Can you work these out from the model? Positions are in its coordinate system, mm. A direction names the side the tool comes from. Coordinates: 2 decimals unless noted, no trailing zeros. Write each loop counter-clockwise with the first axis right and the second up, starting at its lowest first coordinate (ties: lowest second). Pieces come first, ordered by that corner, then holes. Notation, with made-up numbers: M -28.5,55.25 L -12.5,55.25 A20 cw -12.5,59.25 Z; hole C 85,-16.75 d1. An arc over 180 degrees is marked long. Use one line per item in the form item = value. Start each with the question number.
Autodesk Inventor part; units mm, degrees
ref_plane "YZ Plane" through (0, 0, 0) normal (1, 0, 0) x (0, 1, 0)
ref_plane "XZ Plane" through (0, 0, 0) normal (0, 1, 0) x (-1, 0, 0)
ref_plane "XY Plane" through (0, 0, 0) normal (0, 0, 1) x (1, 0, 0)
sketch "Sketch1" plane through (0, 0, 0) normal (0, 1, 0) x (-1, 0, 0)
  line L0 (22, 30) -> (-22, 30)
  line L1 (-22, 30) -> (-22, -30)
  line L2 (-22, -30) -> (22, -30)
  line L3 (22, -30) -> (22, 30)
  line L4 (22, 30) -> (-22, -30) construction
  line L5 (-22, 30) -> (22, -30) construction
  point P0 (0, 0)
  dimension "d0" = 44
  dimension "d1" = 60
extrude "Extrusion1" add sketch "Sketch1" along normal blind 8
sketch "Sketch4" plane through (0, 8, 0) normal (0, 1, 0) x (1, 0, 0)
  circle A0 centre (-17, -24) radius 1.55
  circle A1 centre (17, 24) radius 1.55
  circle A2 centre (17, -24) radius 1.55
  circle A3 centre (-17, 24) radius 1.55
  point P0 (0, 0)
  dimension "d6" = 3.1
  dimension "d7" = 3.1
  dimension "d8" = 3.1
  dimension "d9" = 3.1
  dimension "d10" = 17
  dimension "d11" = 24
  dimension "d12" = 17
  dimension "d13" = 17
  dimension "d14" = 17
  dimension "d15" = 24
  dimension "d16" = 24
  dimension "d17" = 24
hole "Hole1" at (-17, 8, 24) at (-17, 8, -24) at (17, 8, -24) at (17, 8, 24) direction (0, -1, 0) diameter 3.1 depth 8 tip angle 118
sketch "Sketch5" plane through (0, 0, 0) normal (0, -1, 0) x (1, 0, 0)
  line L0 (-12, -18) -> (-22, -18)
  line L1 (-22, -18) -> (-22, -30)
  line L2 (-22, -30) -> (-12, -30)
  line L3 (-12, -30) -> (-12, -18)
  line L4 (22, -18) -> (12, -18)
  line L5 (12, -18) -> (12, -30)
  line L6 (12, -30) -> (22, -30)
  line L7 (22, -30) -> (22, -18)
  line L8 (22, 30) -> (12, 30)
  line L9 (12, 30) -> (12, 18)
  line L10 (12, 18) -> (22, 18)
  line L11 (22, 18) -> (22, 30)
  line L12 (-12, 30) -> (-22, 30)
  line L13 (-22, 30) -> (-22, 18)
  line L14 (-22, 18) -> (-12, 18)
  line L15 (-12, 18) -> (-12, 30)
  line L16 (-22, -30) -> (-22, 30)
  line L17 (22, -30) -> (-22, -30)
  line L18 (22, 30) -> (22, -30)
  line L19 (-22, 30) -> (22, 30)
  point P0 (0, 0)
  dimension "d25" = 10
  dimension "d26" = 12
  dimension "d27" = 10
  dimension "d28" = 12
  dimension "d29" = 10
  dimension "d30" = 12
  dimension "d31" = 10
  dimension "d32" = 12
extrude "Extrusion2" cut sketch "Sketch5" against normal blind 4 contours L3 L2 L1 L0 | L13 L12 L15 L14 | L5 L4 L7 L6 | L8 L11 L10 L9
fillet "Fillet1" radius 3 4 edges at (22, 6, -30) (-22, 6, -30) (22, 6, 30) (-22, 6, 30)
equation "\"d27\" = d25"
equation "\"d28\" = d26"
equation "\"d29\" = d25"
equation "\"d30\" = d26"
equation "\"d31\" = d25"
equation "\"d32\" = d26"
properties part number "motor_driver_support"
1) Will these pins go through, and if not, where does the flat tip stop? pin 1 Ø2 at (y, z) = (2.5, -22.5) entering from +X; pin 2 Ø4.5 at (x, y) = (-19, 1.5) entering from +Z; pin 3 Ø4.5 at (y, z) = (1.5, -22) entering from -X; pin 4 Ø3 at (x, z) = (17, -24) entering from +Y.
2) Suppose I cut it at D-D on x = -14. Please give me the cut outline in (y, z), and give its area (3 significant figures).
3) If we mould it in two halves opening along X, with no side actions, what happens to faces 1 (the face through (-18.537, 5.972, 23.798)), 2 (the face through (-22, 4, 0)), 3 (the face through (15.69, 5.97, 24.83)), 4 (the face through (15.8, 4, -22.6))? For each: +X half, -X half, draft (parallel to the pull), parting line (faces both ways), or undercut.
4) Suppose I cut it at A-A on x = 17. Please give me the cut outline in (y, z).
5) Which directions (+Z, -Z, +X, -X, +Y, -Y) give clear straight access to the entire face, cutting with the end or side of a thin tool? Please do faces 5 (the face through (-17, 2, 18)), 6 (the face through (12, 2, 24)), 7 (the face through (-12, 2, -24)), 8 (the face through (12, 2, -24)).
6) Suppose I cut it at C-C on y = 0.75. Please give me the cut outline in (x, z).
7) Please list where these lines run through material, in increasing order: line 1 (X direction, y = 6.1, z = 24); line 2 (Z direction, x = 17, y = 5.3); line 3 (Z direction, x = 13, y = 3.25).
8) Suppose I cut it at B-B on z = -24. Please give me the cut outline in (x, y).
Computed values:
q1.pin_1 = 12
q1.pin_2 = 18
q1.pin_3 = -12
q1.pin_4 = through
q2.outline = M 0,-18 L 4,-18 L 4,-30 L 8,-30 L 8,30 L 4,30 L 4,18 L 0,18 Z
q2.area = 384 mm²
q3.face_1 = undercut
q3.face_2 = -X half
q3.face_3 = undercut
q3.face_4 = draft
q4.outline = M 0,-18 L 4,-18 L 4,-22.45 L 8,-22.45 L 8,22.45 L 4,22.45 L 4,18 L 0,18 Z; M 4,-30 L 8,-30 L 8,-25.55 L 4,-25.55 Z; M 4,25.55 L 8,25.55 L 8,30 L 4,30 Z
q5.face_5 = +Z, -X, -Y
q5.face_6 = +Z, +X, -Y
q5.face_7 = -Z, -X, -Y
q5.face_8 = -Z, +X, -Y
q6.outline = M -22,-18 L -12,-18 L -12,-30 L 12,-30 L 12,-18 L 22,-18 L 22,18 L 12,18 L 12,30 L -12,30 L -12,18 L -22,18 Z
q7.line_1 = -22 to -18.55, -15.45 to 15.45, 18.55 to 22
q7.line_2 = -30 to -25.55, -22.45 to 22.45, 25.55 to 30
q7.line_3 = -18 to 18
q8.outline = M -22,4 L -18.55,4 L -18.55,8 L -22,8 Z; M -15.45,4 L -12,4 L -12,0 L 12,0 L 12,4 L 15.45,4 L 15.45,8 L -15.45,8 Z; M 18.55,4 L 22,4 L 22,8 L 18.55,8 Z
